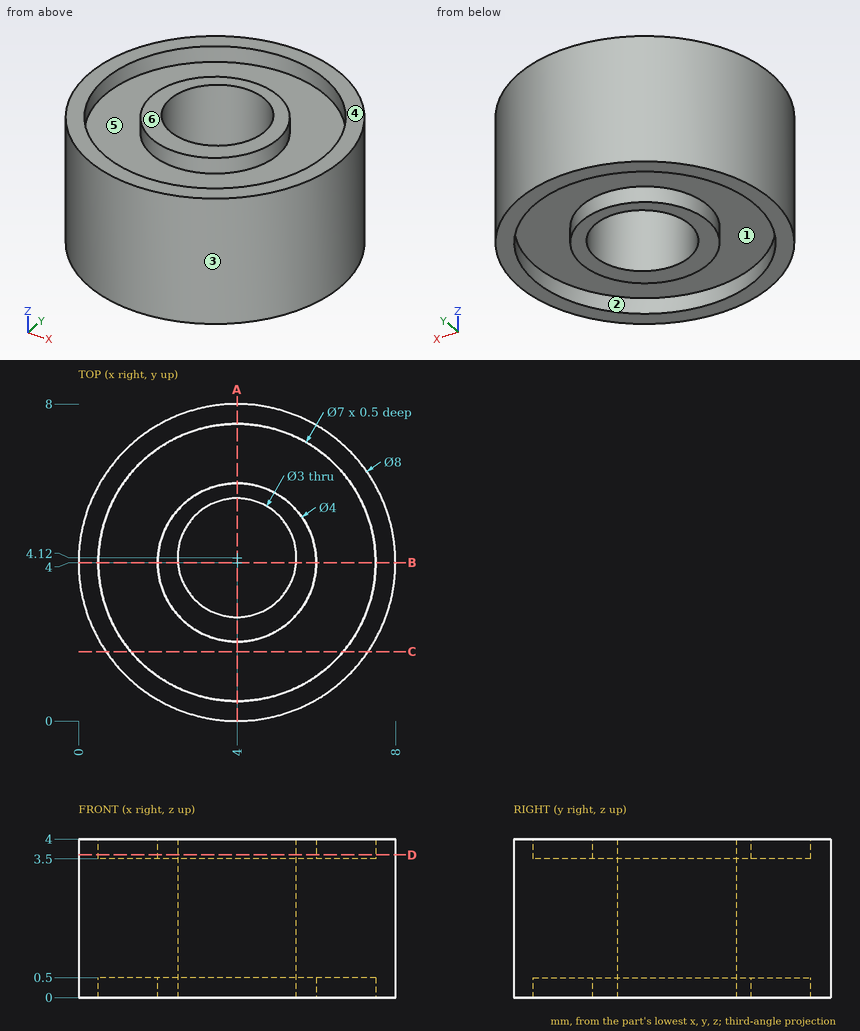
For this review, use the dimensioned drawing (mm, ordinates from the lowest corner) and the shaded views. A direction names the side the tool comes from. Coordinates: 2 decimals unless noted, no trailing zeros. Write each loop counter-clockwise with the first axis right and the second up, starting at its lowest first coordinate (ties: lowest second). Pieces come first, ordered by that corner, then holes. Notation, with made-up numbers: (-23.5, 11.5) -> (-13.5, 11.5) arc R9 ccw to (-13.5, 16.5) -> close; hole circle Ø8 at (-1.75, 51). An arc over 180 degrees is marked (long way). Write each question's results on one line, items separated by ' | '. Start each with the question number.
(1) Tool access review of the marked faces 5 and 6: name each direction out of +Z, -Z, +X, -X, +Y, -Y from which nothing blocks a thin tool from reaching the whole face with its end or side.
(2) The part is to be moulded in two halves that separate along X. For the marked faces 1, 2, 3 and 4, say which applies: pulls with the +X half, pulls with the -X half, needs draft (parallel to the pull), parting line crosses it, or undercut.
(3) Take a section at D-D on z = 3.6. Write out the cut boundary in (x, y).
(4) Take a section at C-C on y = 1.75. Write out the cut boundary in (x, z), and give its area (3 significant figures).
(5) Take a section at B-B on y = 4. Write out the cut boundary in (x, z) (1 decimal).
(6) For line 1 along Y through (x, z) = (4, 0.35); line 2 along X through (y, z) = (3, 0.25) (1 decimal); line 3 along Y through (x, z) = (4, 2.25), list the stretches that pass through material, from the lowest coordinate up. Write a range as from..to.
(7) Take a section at A-A on x = 4. Write out the cut boundary in (y, z), and give its area (3 significant figures).
Results found:
1) face 5: +Z | face 6: +Z, +X, -X, +Y, -Y
2) face 1: undercut | face 2: undercut | face 3: parting line crosses it | face 4: needs draft
3) outline: circle Ø8 at (4, 4); circle Ø4 at (4, 4); hole circle Ø7 at (4, 4); hole circle Ø3 at (4, 4.12)
4) outline: (0.69, 0) -> (1.32, 0) -> (1.32, 0.5) -> (6.68, 0.5) -> (6.68, 0) -> (7.31, 0) -> (7.31, 4) -> (6.68, 4) -> (6.68, 3.5) -> (1.32, 3.5) -> (1.32, 4) -> (0.69, 4) -> close | area: 21.1 mm2
5) outline: (0, 0) -> (0.5, 0) -> (0.5, 0.5) -> (2, 0.5) -> (2, 0) -> (2.5, 0) -> (2.5, 4) -> (2, 4) -> (2, 3.5) -> (0.5, 3.5) -> (0.5, 4) -> (0, 4) -> close; (5.5, 0) -> (6, 0) -> (6, 0.5) -> (7.5, 0.5) -> (7.5, 0) -> (8, 0) -> (8, 4) -> (7.5, 4) -> (7.5, 3.5) -> (6, 3.5) -> (6, 4) -> (5.5, 4) -> close
6) line 1: y = 0..0.5, 2..2.62, 5.62..6, 7.5..8 | line 2: x = 0.1..0.6, 2.3..3, 5..5.7, 7.4..7.9 | line 3: y = 0..2.62, 5.62..8
7) outline: (0, 0) -> (0.5, 0) -> (0.5, 0.5) -> (2, 0.5) -> (2, 0) -> (2.62, 0) -> (2.62, 4) -> (2, 4) -> (2, 3.5) -> (0.5, 3.5) -> (0.5, 4) -> (0, 4) -> close; (5.62, 0) -> (6, 0) -> (6, 0.5) -> (7.5, 0.5) -> (7.5, 0) -> (8, 0) -> (8, 4) -> (7.5, 4) -> (7.5, 3.5) -> (6, 3.5) -> (6, 4) -> (5.62, 4) -> close | area: 17.0 mm2
